The listing builds one solid part. Answer for the finished solid, in the listing's coordinates (mm). A direction names the side the tool comes from. Give positions to 0.01 mm unless a question says otherwise; leave off trailing zeros. Order: outer loops, then holes, each group sorted by start corner. A loop starts at its lowest first (then second) coordinate and runs counter-clockwise, first axis right, second up. Notation, with made-up numbers: (36.5, 61.5) - (43.5, 61.5) arc R35 ccw to (43.5, 94.5) - close; hole circle Ø11 at (73, 22.25). An arc over 180 degrees is marked (long way). Answer in a Markdown table with one row per item. Add a question column.
```python
from build123d import *

# Parameters (mm, degrees)
SKETCH1_W           = 21.844
SKETCH1_H           = 21.844
BOSS_EXTRUDE2_DEPTH = 50.8
SKETCH2_W           = 25.4
SKETCH2_H           = 25.4
BOSS_EXTRUDE3_DEPTH = 6.35
SKETCH4_R           = 2.794
CUT_EXTRUDE2_DEPTH  = 67.198133271
SKETCH5_R           = 6.604
CUT_EXTRUDE3_DEPTH  = 67.33394917


with BuildPart() as part:
    # Sketch1 → Boss-Extrude2 (new body)
    with BuildSketch(Plane.XY):
        with Locations((10.922, 10.922)):
            Rectangle(SKETCH1_W, SKETCH1_H)
    extrude(amount=BOSS_EXTRUDE2_DEPTH)

    # Sketch2 → Boss-Extrude3 (add)
    with BuildSketch(Plane.XY.offset(50.8)):
        with Locations((11.1125, 10.7315)):
            Rectangle(SKETCH2_W, SKETCH2_H)
    extrude(amount=BOSS_EXTRUDE3_DEPTH)

    # Sketch4 → Cut-Extrude2 (cut, through all)
    with BuildSketch(Plane.ZY):
        with Locations((38.1, 10.922)):
            Circle(SKETCH4_R)
        with Locations((12.7, 10.922)):
            Circle(SKETCH4_R)
    extrude(amount=-CUT_EXTRUDE2_DEPTH, mode=Mode.SUBTRACT)

    # Sketch5 → Cut-Extrude3 (cut, through all)
    with BuildSketch(Plane(origin=(0, 21.844, 0), x_dir=(1, 0, 0), z_dir=(0, 1, 0))):
        with Locations(Location((10.922, -25.4, 0), (0, 0, 270))):
            Circle(SKETCH5_R)
    extrude(amount=-CUT_EXTRUDE3_DEPTH, mode=Mode.SUBTRACT)

    # Chamfer2
    # the kernel refuses this chamfer: 2.54 mm, written as the material it takes off along each edge
    with BuildSketch(Plane(origin=(20.150666667, 20.150666667, 1.693333333), x_dir=(0, -0.7071067811865474, -0.7071067811865477), z_dir=(0.5773502691896258, 0.5773502691896258, -0.5773502691896255)), Plane(origin=(1.693333333, 20.150666667, 1.693333333), x_dir=(-0.7071067811865476, -0.7071067811865476, 0), z_dir=(-0.5773502691896257, 0.5773502691896257, -0.5773502691896258)), Plane(origin=(20.150666667, 1.693333333, 1.693333333), x_dir=(0, -0.7071067811865476, 0.7071067811865474), z_dir=(0.5773502691896257, -0.5773502691896256, -0.5773502691896257))) as chamfer2_piece_1:
        Polygon((-1.796051224, 1.036950658), (1.796051224, 1.036950658), (0, -2.073901316), align=None)
    extrude(amount=3.226233304, mode=Mode.SUBTRACT)
    with BuildSketch(Plane(origin=(1.693333333, 1.693333333, 1.693333333), x_dir=(0.7071067811865476, 0, -0.7071067811865474), z_dir=(-0.5773502691896255, -0.5773502691896256, -0.5773502691896261))) as chamfer2_piece_2:
        Polygon((-1.796051224, -1.036950658), (1.796051224, -1.036950658), (0, 2.073901316), align=None)
    extrude(amount=3.226233304, mode=Mode.SUBTRACT)
    with BuildSketch(Plane(origin=(-1.5875, 29.963574789, 57.15), x_dir=(-0.027495876610586334, 0, -0.9996219169112968), z_dir=(0, -1, 0)), Plane(origin=(-8.119574789, -1.9685, 57.15), x_dir=(0, -0.02749587661058642, -0.9996219169112968), z_dir=(1, 0, 0)), Plane(origin=(23.8125, -8.500574789, 57.15), x_dir=(0.02749587661058591, 0, -0.9996219169112968), z_dir=(0, 1, 0))) as chamfer2_piece_3:
        with BuildLine():
            Line((2.612829916, 0), (-0.143629773, 2.608879196))
            Line((-0.143629773, 2.608879196), (-0.194410567, 2.607482405))
            ThreePointArc((-0.194410567, 2.607482405), (-0.086688237, 1.304030487), (-0.050780793, -0.001396791))
            Line((-0.050780793, -0.001396791), (0.001396791, -0.050780793))
            ThreePointArc((0.001396791, -0.050780793), (1.306824068, -0.01487335), (2.614226706, -0.050780793))
            Line((2.614226706, -0.050780793), (2.612829916, 0))
        make_face()
    extrude(amount=38.464149579, mode=Mode.SUBTRACT)
    with BuildSketch(Plane(origin=(30.344574789, 23.4315, 57.15), x_dir=(0, -0.9996219169112966, 0.027495876610587302), z_dir=(-1, 0, 0))) as chamfer2_piece_4:
        with BuildLine():
            Line((2.612829916, 0), (-0.143629773, -2.608879196))
            Line((-0.143629773, -2.608879196), (-0.194410567, -2.607482405))
            ThreePointArc((-0.194410567, -2.607482405), (-0.086688237, -1.304030487), (-0.050780793, 0.001396791))
            Line((-0.050780793, 0.001396791), (0.001396791, 0.050780793))
            ThreePointArc((0.001396791, 0.050780793), (1.306824068, 0.01487335), (2.614226706, 0.050780793))
            Line((2.614226706, 0.050780793), (2.612829916, 0))
        make_face()
    extrude(amount=38.464149579, mode=Mode.SUBTRACT)
    with BuildSketch(Plane(origin=(21.844, 10.922, 38.1), x_dir=(0, 0, 1), z_dir=(0, -1, 0))) as chamfer2_piece_5:
        with BuildLine():
            Line((5.405842049, -0.071842049), (2.722157951, 2.611842049))
            Line((2.722157951, 2.611842049), (2.671357951, 2.611842049))
            ThreePointArc((2.671357951, 2.611842049), (2.7432, 1.305921024), (2.7432, 0))
            Line((2.7432, 0), (2.794, -0.0508))
            ThreePointArc((2.794, -0.0508), (4.099921024, -0.0508), (5.405842049, -0.122642049))
            Line((5.405842049, -0.122642049), (5.405842049, -0.071842049))
        make_face()
    revolve(axis=Axis((21.844, 10.922, 38.1), (-1, 0, 0)), mode=Mode.SUBTRACT)
    with BuildSketch(Plane(origin=(0, 10.922, 38.1), x_dir=(0, 0, 1), z_dir=(0, -1, 0))) as chamfer2_piece_6:
        with BuildLine():
            Line((5.405842049, 0.071842049), (2.722157951, -2.611842049))
            Line((2.722157951, -2.611842049), (2.671357951, -2.611842049))
            ThreePointArc((2.671357951, -2.611842049), (2.7432, -1.305921024), (2.7432, 0))
            Line((2.7432, 0), (2.794, 0.0508))
            ThreePointArc((2.794, 0.0508), (4.099921024, 0.0508), (5.405842049, 0.122642049))
            Line((5.405842049, 0.122642049), (5.405842049, 0.071842049))
        make_face()
    revolve(axis=Axis((0, 10.922, 38.1), (-1, 0, 0)), mode=Mode.SUBTRACT)
    with BuildSketch(Plane(origin=(21.844, 10.922, 12.7), x_dir=(0, 0, 1), z_dir=(0, -1, 0))) as chamfer2_piece_7:
        with BuildLine():
            Line((5.405842049, -0.071842049), (2.722157951, 2.611842049))
            Line((2.722157951, 2.611842049), (2.671357951, 2.611842049))
            ThreePointArc((2.671357951, 2.611842049), (2.7432, 1.305921024), (2.7432, 0))
            Line((2.7432, 0), (2.794, -0.0508))
            ThreePointArc((2.794, -0.0508), (4.099921024, -0.0508), (5.405842049, -0.122642049))
            Line((5.405842049, -0.122642049), (5.405842049, -0.071842049))
        make_face()
    revolve(axis=Axis((21.844, 10.922, 12.7), (-1, 0, 0)), mode=Mode.SUBTRACT)
    with BuildSketch(Plane(origin=(0, 10.922, 12.7), x_dir=(0, 0, 1), z_dir=(0, -1, 0))) as chamfer2_piece_8:
        with BuildLine():
            Line((5.405842049, 0.071842049), (2.722157951, -2.611842049))
            Line((2.722157951, -2.611842049), (2.671357951, -2.611842049))
            ThreePointArc((2.671357951, -2.611842049), (2.7432, -1.305921024), (2.7432, 0))
            Line((2.7432, 0), (2.794, 0.0508))
            ThreePointArc((2.794, 0.0508), (4.099921024, 0.0508), (5.405842049, 0.122642049))
            Line((5.405842049, 0.122642049), (5.405842049, 0.071842049))
        make_face()
    revolve(axis=Axis((0, 10.922, 12.7), (-1, 0, 0)), mode=Mode.SUBTRACT)
    with BuildSketch(Plane(origin=(10.922, 0, 25.4), x_dir=(0, 0, 1), z_dir=(-1, 0, 0))) as chamfer2_piece_9:
        with BuildLine():
            Line((9.215842049, -0.071842049), (6.532157951, 2.611842049))
            Line((6.532157951, 2.611842049), (6.481357951, 2.611842049))
            ThreePointArc((6.481357951, 2.611842049), (6.5532, 1.305921024), (6.5532, 0))
            Line((6.5532, 0), (6.604, -0.0508))
            ThreePointArc((6.604, -0.0508), (7.909921024, -0.0508), (9.215842049, -0.122642049))
            Line((9.215842049, -0.122642049), (9.215842049, -0.071842049))
        make_face()
    revolve(axis=Axis((10.922, 0, 25.4), (0, 1, 0)), mode=Mode.SUBTRACT)
    with BuildSketch(Plane(origin=(10.922, 21.844, 25.4), x_dir=(0, 0, 1), z_dir=(-1, 0, 0))) as chamfer2_piece_10:
        with BuildLine():
            Line((9.215842049, 0.071842049), (6.532157951, -2.611842049))
            Line((6.532157951, -2.611842049), (6.481357951, -2.611842049))
            ThreePointArc((6.481357951, -2.611842049), (6.5532, -1.305921024), (6.5532, 0))
            Line((6.5532, 0), (6.604, 0.0508))
            ThreePointArc((6.604, 0.0508), (7.909921024, 0.0508), (9.215842049, 0.122642049))
            Line((9.215842049, 0.122642049), (9.215842049, 0.071842049))
        make_face()
    revolve(axis=Axis((10.922, 21.844, 25.4), (0, 1, 0)), mode=Mode.SUBTRACT)
    with BuildSketch(Plane(origin=(28.376074789, 21.844, 0), x_dir=(0, 0.027495876610585925, 0.9996219169112968), z_dir=(-1, 0, 0)), Plane(origin=(21.844, -6.532074789, 0), x_dir=(0.027495876610585925, 0, 0.9996219169112968), z_dir=(0, 1, 0)), Plane(origin=(-6.532074789, 0, 0), x_dir=(0, -0.027495876610586376, 0.9996219169112968), z_dir=(1, 0, 0)), Plane(origin=(0, 28.376074789, 0), x_dir=(-0.027495876610586376, 0, 0.9996219169112968), z_dir=(0, -1, 0))) as chamfer2_piece_11:
        with BuildLine():
            Line((2.612829916, 0), (-0.143629773, -2.608879196))
            Line((-0.143629773, -2.608879196), (-0.194410567, -2.607482405))
            ThreePointArc((-0.194410567, -2.607482405), (-0.086688237, -1.304030487), (-0.050780793, 0.001396791))
            Line((-0.050780793, 0.001396791), (0.001396791, 0.050780793))
            ThreePointArc((0.001396791, 0.050780793), (1.306824068, 0.01487335), (2.614226706, 0.050780793))
            Line((2.614226706, 0.050780793), (2.612829916, 0))
        make_face()
    extrude(amount=34.908149579, mode=Mode.SUBTRACT)
    with BuildSketch(Plane(origin=(0, 21.844, -6.532074789), x_dir=(0.9996219169112968, 0.027495876610585935, 0), z_dir=(0, 0, 1)), Plane(origin=(21.844, 21.844, -6.532074789), x_dir=(0.02749587661058595, -0.9996219169112968, 0), z_dir=(0, 0, 1)), Plane(origin=(21.844, 0, -6.532074789), x_dir=(-0.9996219169112966, -0.0274958766105864, 0), z_dir=(0, 0, 1))) as chamfer2_piece_12:
        with BuildLine():
            Line((2.612829916, 0), (-0.143629773, -2.608879196))
            Line((-0.143629773, -2.608879196), (-0.194410567, -2.607482405))
            ThreePointArc((-0.194410567, -2.607482405), (-0.086688237, -1.304030487), (-0.050780793, 0.001396791))
            Line((-0.050780793, 0.001396791), (0.001396791, 0.050780793))
            ThreePointArc((0.001396791, 0.050780793), (1.306824068, 0.01487335), (2.614226706, 0.050780793))
            Line((2.614226706, 0.050780793), (2.612829916, 0))
        make_face()
    extrude(amount=57.332074789, mode=Mode.SUBTRACT)
    with BuildSketch(Plane(origin=(0, 0, -6.532074789), x_dir=(0.9996219169112966, -0.02749587661058636, 0), z_dir=(0, 0, 1))) as chamfer2_piece_13:
        with BuildLine():
            Line((2.612829916, 0), (-0.143629773, 2.608879196))
            Line((-0.143629773, 2.608879196), (-0.194410567, 2.607482405))
            ThreePointArc((-0.194410567, 2.607482405), (-0.086688237, 1.304030487), (-0.050780793, -0.001396791))
            Line((-0.050780793, -0.001396791), (0.001396791, -0.050780793))
            ThreePointArc((0.001396791, -0.050780793), (1.306824068, -0.01487335), (2.614226706, -0.050780793))
            Line((2.614226706, -0.050780793), (2.612829916, 0))
        make_face()
    extrude(amount=57.332074789, mode=Mode.SUBTRACT)


solid = part.part
```
(1) Straight lines are drawn through the part: line 1 (Z direction, x = 18.5, y = 11.5); line 2 (X direction, y = 7.5, z = 25.4); line 3 (Z direction, x = 16, y = 12.25). For each, find the intervals that lie inside material, in ascending order.
(2) For faces 4 (the face through (1.288, 20.592, 26.332)), 5 (the face through (11, 0, 10)), 6 (the face through (20.274, 20.071, 1.737)), 7 (the face through (21.844, 11, 26)), 8 (the face through (22, 11, 50.8)), determine the directions among +Z, -Z, +X, -X, +Y, -Y from which every point of the face is accessible in a straight line to the end or side of a thin tool.
(3) Find section A-A, the plane z = 38.1. Write down the section's boundary in (x, y).
(4) Find section D-D, the plane z = 47. Write down the section's boundary in (x, y).
(5) Find section B-B, the plane y = 5. Write down the section's boundary in (x, z).
(6) Each of these flat-tipped pins is pushed along its axis until it touches: P1, Ø6.5, axis at y = 10.922, z = 38.1, coming from the +X side; P2, Ø13.5, axis at x = 13.5, z = 40, coming from the -Y side; P3, Ø12, axis at x = 12.5, z = 8.5, coming from the +Y side. Where does it stop, or does it pass through?
(7) Find section C-C, the plane x = 13.5. Give the number of separate pieces and of enclosed holes in the cut face, plus the area to 3 significant figures.
(8) The mould has two halves that part along Z. Classify faces 1 (the face through (11, 11, 57.15)), 2 (the face through (19.43, 8.07, 12.07)), 3 (the face through (11, 21.844, 42)): +Z half, -Z half, draft (parallel to the pull), parting line (faces both ways), or undercut.
Answer key:
| question | item | result |
|---|---|---|
| 1 | line 1 | 0 to 9.97, 15.43 to 35.37, 40.83 to 57.15 |
| 1 | line 2 | 0 to 4.32, 17.53 to 21.84 |
| 1 | line 3 | 0 to 10.24, 15.16 to 21.18, 29.62 to 35.64, 40.56 to 57.15 |
| 2 | face 4 | -Z, -X, +Y |
| 2 | face 5 | -Z, +X, -X, -Y |
| 2 | face 6 | -Z, +X, +Y |
| 2 | face 7 | -Z, +X, +Y, -Y |
| 2 | face 8 | -Z |
| 3 | outline | (0, 2.54) - (2.54, 0) - (19.3, 0) - (21.84, 2.54) - (21.84, 5.59) - (19.3, 8.13) - (2.54, 8.13) - (0, 5.59) - close; (0, 16.26) - (2.54, 13.72) - (19.3, 13.72) - (21.84, 16.26) - (21.84, 19.3) - (19.3, 21.84) - (2.54, 21.84) - (0, 19.3) - close |
| 4 | outline | (0, 2.54) - (2.54, 0) - (19.3, 0) - (21.84, 2.54) - (21.84, 19.3) - (19.3, 21.84) - (2.54, 21.84) - (0, 19.3) - close |
| 5 | outline | (-1.59, 50.8) - (0, 50.8) - (0, 2.54) - (2.54, 0) - (19.3, 0) - (21.84, 2.54) - (21.84, 50.8) - (23.81, 50.8) - (23.81, 54.61) - (21.27, 57.15) - (0.95, 57.15) - (-1.59, 54.61) - close; hole circle Ø13.21 at (10.92, 25.4) |
| 6 | P1 | x = 19.76 |
| 6 | P2 | y = 0 |
| 6 | P3 | y = 21.84 |
| 7 | separate pieces | 2 |
| 7 | enclosed holes | 2 |
| 7 | area | 930 mm² |
| 8 | face 1 | +Z half |
| 8 | face 2 | undercut |
| 8 | face 3 | draft |
